```python
from build123d import *

# Parameters (mm, degrees)
F1_DEPTH = 133.35


with BuildPart() as f1:
    # F0 (on Top) → F1 (new body)
    with BuildSketch(Plane.XY):
        with BuildLine():
            Line((-0.059343, 41.325617), (-0.059343, -9.474383))
            Line((-0.059343, -9.474383), (41.215657, -9.474383))
            Line((41.215657, -9.474383), (41.215657, -0.584383))
            ThreePointArc((41.215657, -0.584383), (29.351853, 29.011377), (-0.059343, 41.325617))
        make_face()
    extrude(amount=F1_DEPTH)

    # F2: F1 across face


with BuildPart() as f1_1:
    add(f1.part)
    add(f1.part.mirror(Plane(origin=(-0.059343, 15.925617, 66.675), x_dir=(0, -1, 0), z_dir=(-1, 0, 0))))


solid = f1_1.part
```
CAD build for the part. Positions are in the model's coordinates, mm. Round coordinates to 2 decimals unless told otherwise and drop trailing zeros. Order: outer loops, then holes, each group sorted by start corner. A loop starts at its lowest first (then second) coordinate and runs counter-clockwise, first axis right, second up.
Q1. Slice it at C-C (y = 15). Write the cut outline in (x, z).
Q2. Drop flat-ended pins along their axis: pin 1 (2 mm diameter, centred on y = 14.5, z = 51, fed in from +X); pin 2 (1 mm diameter, centred on x = -29.5, z = 96, fed in from +Y); pin 3 (5 mm diameter, centred on x = 10, z = 15, fed in from +Y). Give the stop position or say it passes through.
Q3. Wall check: L1, parallel to X at y = -6.5, z = 93.5; L2, parallel to Y at x = 19.5, z = 94.5; L3, parallel to Y at x = -9.5, z = 101. Give the ranges that are in metal, low to high.
Q4. Slice it at A-A (z = 13). Write the cut outline in (x, y), and give its area (3 significant figures).
Q5. Slice it at B-B (x = 26). Write the cut outline in (y, z).
Results below:
1. outline: (-38.54, 0) - (38.42, 0) - (38.42, 133.35) - (-38.54, 133.35) - close
2. pin 1: stops at x = 38.97
2. pin 2: stops at y = 29.48
2. pin 3: stops at y = 40.63
3. L1: x = -41.33 to 41.22
3. L2: y = -9.47 to 36.4
3. L3: y = -9.47 to 40.23
4. outline: (-41.33, -9.47) - (41.22, -9.47) - (41.22, -0.58) arc R41.28 ccw to (-0.06, 41.33) arc R41.28 ccw to (-41.33, -0.58) - close
4. area: 3,460 mm2
5. outline: (-9.47, 0) - (32.06, 0) - (32.06, 133.35) - (-9.47, 133.35) - close
